```python
from build123d import *

# Parameters (mm, degrees)
BOSS_EXTRUDE2_DEPTH = 2
SKETCH3_R           = 5
BOSS_EXTRUDE3_DEPTH = 5


with BuildPart() as part:
    # Sketch1 → Boss-Extrude2 (new body)
    with BuildSketch(Plane(origin=(0, 0, 0), x_dir=(1, 0, 0), z_dir=(0, 1, 0))):
        with BuildLine():
            Line((-55, -7.5), (55, -7.5))
            ThreePointArc((55, -7.5), (58.535533906, -6.035533906), (60, -2.5))
            Line((60, -2.5), (60, 2.5))
            ThreePointArc((60, 2.5), (58.535533906, 6.035533906), (55, 7.5))
            Line((55, 7.5), (-55, 7.5))
            ThreePointArc((-55, 7.5), (-58.535533906, 6.035533906), (-60, 2.5))
            Line((-60, 2.5), (-60, -2.5))
            ThreePointArc((-60, -2.5), (-58.535533906, -6.035533906), (-55, -7.5))
        make_face()
    extrude(amount=BOSS_EXTRUDE2_DEPTH)

    # Sketch3 → Boss-Extrude3 (add)
    with BuildSketch(Plane(origin=(0, 2, 0), x_dir=(1, 0, 0), z_dir=(0, 1, 0))):
        with Locations((52, 0)):
            Circle(SKETCH3_R)
        with Locations((-52, 0)):
            Circle(SKETCH3_R)
    extrude(amount=BOSS_EXTRUDE3_DEPTH)


solid = part.part
```
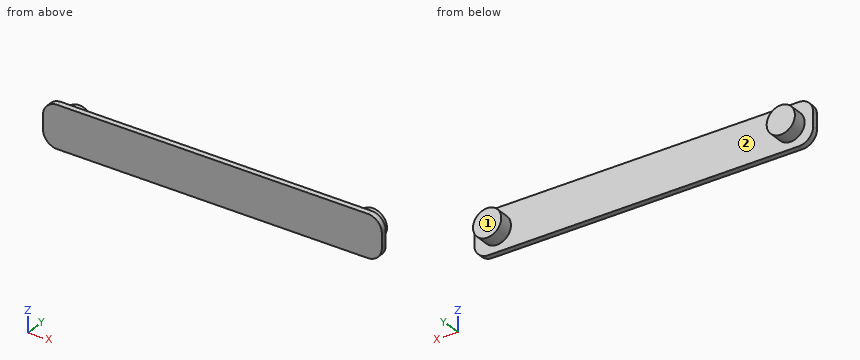
Could you check a few things on this model? Use its own coordinates, in mm. Face numbers are marked on the shaded views. Round coordinates to 2 decimals unless told otherwise and drop trailing zeros. Write each loop counter-clockwise with the first axis right and the second up, starting at its lowest first coordinate (ties: lowest second). Pieces come first, ordered by that corner, then holes. Notation, with made-up numbers: M 86.25,23 L 91.25,23 A17 ccw 91.25,40 Z; hole C -31,-2 d9. An arc over 180 degrees is marked long. Write each question's results on one line, items separated by ' | '. Start each with the question number.
1. Imagine slicing it at C-C on y = 3.5. List the corners of the cut face in (x, z) for me.
2. Thinking about a two-plate mould opening in X: for the marked faces 1 and 2, which applies, +X half, -X half, draft (parallel to the pull), parting line (faces both ways), or undercut?
3. I'm going to push flat-ended pins straight in: pin 1 Ø3 at (y, z) = (2.5, 5) entering from +X; pin 2 Ø4.5 at (x, z) = (-10, 1) entering from +Y; pin 3 Ø2 at (y, z) = (5.5, 4) entering from -X. Where does each tip first touch, or does it pass through?
4. Imagine slicing it at A-A on z = 0. List the corners of the cut face in (x, y) for me, and give its area (3 significant figures).
5. I need wall thicknesses on L1, parallel to X at y = 5, z = 0; L2, parallel to Y at x = 40.5, z = 0; L3, parallel to X at y = 5, z = -3.75. Which ranges of each line are inside material? Lowest first, please. Write a range as from..to.
6. Imagine slicing it at D-D on x = -11. List the corners of the cut face in (y, z) for me, and give its area (3 significant figures).
7. Imagine slicing it at B-B on x = -52. List the corners of the cut face in (y, z) for me.
Result sheet:
1) outline: C -52,0 d10; C 52,0 d10
2) face 1: draft | face 2: undercut
3) pin 1: stops at x = 59.88 | pin 2: stops at y = 2 | pin 3: stops at x = -56
4) outline: M -60,0 L 60,0 L 60,2 L 57,2 L 57,7 L 47,7 L 47,2 L -47,2 L -47,7 L -57,7 L -57,2 L -60,2 Z | area: 340 mm^2
5) L1: x = -57..-47, 47..57 | L2: y = 0..2 | L3: x = -55.31..-48.69, 48.69..55.31
6) outline: M 0,-7.5 L 2,-7.5 L 2,7.5 L 0,7.5 Z | area: 30.0 mm^2
7) outline: M 0,-7.5 L 2,-7.5 L 2,-5 L 7,-5 L 7,5 L 2,5 L 2,7.5 L 0,7.5 Z
